from build123d import *

# Parameters (mm, degrees)
SKETCH_1_W           = 98.5
SKETCH_1_H           = 65
EXTRUDE_1_DEPTH      = 3.5
SKETCH_2_W           = 98.5
SKETCH_2_H           = 65
SKETCH_2_W_2         = 94.5
SKETCH_2_H_2         = 62
EXTRUDE_2_DEPTH      = 19
SKETCH_9_R           = 1.75
CUT_EXTRUDE_7_DEPTH  = 64.151108462
SKETCH_10_R          = 2.25
SKETCH_10_R_2        = 1.75
EXTRUDE_6_DEPTH      = 19
SKETCH_11_W          = 8.5
SKETCH_11_H          = 15.9
CUT_EXTRUDE_8_DEPTH  = 7
SKETCH_12_W          = 50
SKETCH_12_H          = 6
CUT_EXTRUDE_9_DEPTH  = 7
SKETCH_13_R          = 3.05
CUT_EXTRUDE_10_DEPTH = 3


with BuildPart() as part:
    # 草图1 → 凸台-拉伸1 (new body)
    with BuildSketch(Plane(origin=(0, 0, 0), x_dir=(1, 0, 0), z_dir=(0, 1, 0))):
        Rectangle(SKETCH_1_W, SKETCH_1_H)
    extrude(amount=EXTRUDE_1_DEPTH)

    # 草图2 → 凸台-拉伸2 (add)
    with BuildSketch(Plane(origin=(0, 0, 0), x_dir=(-1, 0, 0), z_dir=(0, -1, 0))):
        Rectangle(SKETCH_2_W, SKETCH_2_H)
        Rectangle(SKETCH_2_W_2, SKETCH_2_H_2, mode=Mode.SUBTRACT)
    extrude(amount=EXTRUDE_2_DEPTH)

    # 草图9 → 切除-拉伸7 (cut, through all)
    with BuildSketch(Plane(origin=(0, 3.5, 0), x_dir=(1, 0, 0), z_dir=(0, 1, 0))):
        with Locations(Location((46.25, 29.5, 0), (0, 0, 270))):
            Circle(SKETCH_9_R)
        with Locations(Location((46.25, -29.5, 0), (0, 0, 270))):
            Circle(SKETCH_9_R)
        with Locations(Location((-37.117, 29.5, 0), (0, 0, 270))):
            Circle(SKETCH_9_R)
        with Locations(Location((-37.117, -29.5, 0), (0, 0, 270))):
            Circle(SKETCH_9_R)
    extrude(amount=-CUT_EXTRUDE_7_DEPTH, mode=Mode.SUBTRACT)

    # 草图10 → 凸台-拉伸6 (add, through all)
    # profile 1 of 4: a face of its own
    with BuildSketch(Plane(origin=(0, 0, 0), x_dir=(-1, 0, 0), z_dir=(0, -1, 0))):
        with Locations((-46.25, 29.5)):
            Circle(SKETCH_10_R)
        with Locations(Location((-46.25, 29.5, 0), (0, 0, 270))):
            Circle(SKETCH_10_R_2, mode=Mode.SUBTRACT)
    # profile 2 of 4: a face of its own
    with BuildSketch(Plane(origin=(0, 0, 0), x_dir=(-1, 0, 0), z_dir=(0, -1, 0))):
        with Locations((37.117, 29.5)):
            Circle(SKETCH_10_R)
        with Locations(Location((37.117, 29.5, 0), (0, 0, 270))):
            Circle(SKETCH_10_R_2, mode=Mode.SUBTRACT)
    # profile 3 of 4: a face of its own
    with BuildSketch(Plane(origin=(0, 0, 0), x_dir=(-1, 0, 0), z_dir=(0, -1, 0))):
        with Locations((-46.25, -29.5)):
            Circle(SKETCH_10_R)
        with Locations(Location((-46.25, -29.5, 0), (0, 0, 270))):
            Circle(SKETCH_10_R_2, mode=Mode.SUBTRACT)
    # profile 4 of 4: a face of its own
    with BuildSketch(Plane(origin=(0, 0, 0), x_dir=(-1, 0, 0), z_dir=(0, -1, 0))):
        with Locations((37.117, -29.5)):
            Circle(SKETCH_10_R)
        with Locations(Location((37.117, -29.5, 0), (0, 0, 270))):
            Circle(SKETCH_10_R_2, mode=Mode.SUBTRACT)
    extrude(amount=EXTRUDE_6_DEPTH)

    # 草图11 → 切除-拉伸8 (cut)
    with BuildSketch(Plane(origin=(0, -19, 0), x_dir=(-1, 0, 0), z_dir=(0, -1, 0))):
        with Locations((45, 24.55)):
            Rectangle(SKETCH_11_W, SKETCH_11_H)
    extrude(amount=-CUT_EXTRUDE_8_DEPTH, mode=Mode.SUBTRACT)

    # 草图12 → 切除-拉伸9 (cut)
    with BuildSketch(Plane(origin=(49.25, 0, 0), x_dir=(0, 0, -1), z_dir=(1, 0, 0))):
        with Locations((0, -19)):
            Rectangle(SKETCH_12_W, SKETCH_12_H)
    extrude(amount=-CUT_EXTRUDE_9_DEPTH, mode=Mode.SUBTRACT)

    # 草图13 → 切除-拉伸10 (cut)
    with BuildSketch(Plane(origin=(0, 3.5, 0), x_dir=(1, 0, 0), z_dir=(0, 1, 0))):
        with Locations((-37.117, 29.5)):
            Circle(SKETCH_13_R)
        with Locations((46.25, 29.5)):
            Circle(SKETCH_13_R)
        with Locations((46.25, -29.5)):
            Circle(SKETCH_13_R)
        with Locations((-37.117, -29.5)):
            Circle(SKETCH_13_R)
    extrude(amount=-CUT_EXTRUDE_10_DEPTH, mode=Mode.SUBTRACT)


solid = part.part
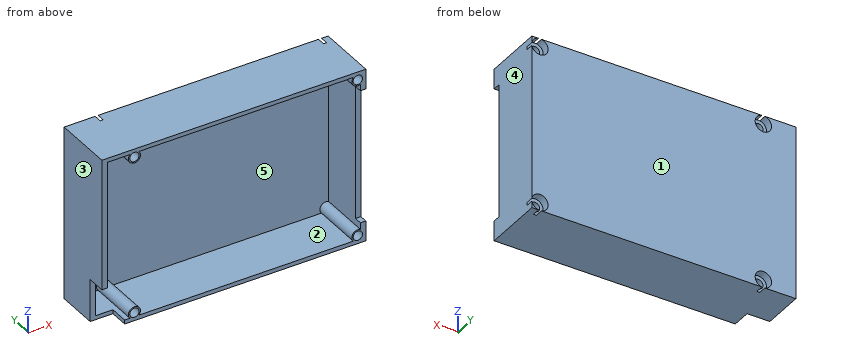
CAD build for the part. Positions are in the model's coordinates, mm. Face numbers are marked on the shaded views. A direction names the side the tool comes from. Give positions to 0.01 mm unless a question says otherwise; leave off trailing zeros. Order: outer loops, then holes, each group sorted by start corner. A loop starts at its lowest first (then second) coordinate and runs counter-clockwise, first axis right, second up. Notation, with made-up numbers: (20, 75) -> (73, 75) arc R23 cw to (73, 90) -> close; hole circle Ø6 at (7, 40.5). An arc over 180 degrees is marked (long way). Return JSON: item names as keys, results as strings.
Q1. Which spindle directions (+Z, -Z, +X, -X, +Y, -Y) get a long thin tool onto all of the face, cutting with end or side? Do the marked faces 4 and 5. Say none if no direction does.
Working result:
{"face 4": "+Z, -Z, +X, +Y, -Y", "face 5": "-Y"}
Q2. Drill centre lines: line 1 (X direction, y = -4, z = -29.5); line 2 (X direction, y = -3.25, z = 20.5); line 3 (Z direction, x = 3.5, y = -3.5). Where is each one in solid material? Low to high.
Working result:
{"line 1": "-49.25 to -47.25, -39.37 to -38.87, -35.37 to -34.87, 44 to 44.5, 48 to 49.25", "line 2": "-49.25 to -47.25, 47.25 to 49.25", "line 3": "-32.5 to -31, 31 to 32.5"}
Q3. Flat gauge pins, fed straight in: pin 1 (0.6 mm diameter, centred on x = 48.5, z = 10, fed in from -Y); pin 2 (1.6 mm diameter, centred on y = -15.5, z = -32, fed in from -X); pin 3 (1.8 mm diameter, centred on x = 47, z = 30.5, fed in from +Y). Where does each tip first touch, or does it go through?
Working result:
{"pin 1": "y = -16", "pin 2": "x = -40.75", "pin 3": "y = 0.5"}
Q4. Saw through at B-B (x = -42.5). Write the cut outline in (y, z), then the cut area to 3 significant figures.
Working result:
{"outline": "(-19, 31) -> (0, 31) -> (0, -31) -> (-12, -31) -> (-12, -32.5) -> (3.5, -32.5) -> (3.5, 32.5) -> (-19, 32.5) -> close", "area": "274 mm²"}
Q5. Saw through at D-D (y = -5.5). Write the cut outline in (x, z).
Working result:
{"outline": "(-49.25, -32.5) -> (49.25, -32.5) -> (49.25, 32.5) -> (-49.25, 32.5) -> close; hole (-47.25, -31) -> (-38.79, -31) arc R2.25 cw (long way) to (-35.44, -31) -> (44.57, -31) arc R2.25 cw to (47.25, -27.48) -> (47.25, 27.48) arc R2.25 cw to (44.57, 31) -> (-35.44, 31) arc R2.25 cw (long way) to (-38.79, 31) -> (-47.25, 31) -> close; hole circle Ø3.5 at (-37.12, -29.5); hole circle Ø3.5 at (-37.12, 29.5); hole circle Ø3.5 at (46.25, -29.5); hole circle Ø3.5 at (46.25, 29.5)"}
Q6. Saw through at C-C (y = -13.75). Write the cut outline in (x, z).
Working result:
{"outline": "(-49.25, -16.6) -> (-47.25, -16.6) -> (-47.25, 31) -> (-38.79, 31) arc R2.25 ccw (long way) to (-35.44, 31) -> (44.57, 31) arc R2.25 ccw to (47.25, 27.48) -> (47.25, -27.48) arc R2.25 ccw to (44.57, -31) -> (-35.44, -31) arc R2.25 ccw (long way) to (-38.79, -31) -> (-40.75, -31) -> (-40.75, -32.5) -> (49.25, -32.5) -> (49.25, 32.5) -> (-49.25, 32.5) -> close; hole circle Ø3.5 at (-37.12, -29.5); hole circle Ø3.5 at (-37.12, 29.5); hole circle Ø3.5 at (46.25, -29.5); hole circle Ø3.5 at (46.25, 29.5)"}
Q7. Mould opens along X. For the marked faces 1, 2 and 3 say: pulls with the +X half, pulls with the -X half, needs draft (parallel to the pull), parting line crosses it, or undercut.
Working result:
{"face 1": "needs draft", "face 2": "undercut", "face 3": "pulls with the -X half"}
Q8. Saw through at A-A (z = 9.5). Write the cut outline in (x, y).
Working result:
{"outline": "(-49.25, -19) -> (-47.25, -19) -> (-47.25, 0) -> (47.25, 0) -> (47.25, -16) -> (49.25, -16) -> (49.25, 3.5) -> (-49.25, 3.5) -> close"}
